```python
from build123d import *

# Parameters (mm, degrees)
SKETCH_W     = 80
SKETCH_H     = 9.5
PAD_DEPTH    = 10
SKETCH001_W  = 70
SKETCH001_H  = 25
POCKET_DEPTH = 6.3
SKETCH002_R  = 0.8
HOLE_DEPTH   = 10.001


with BuildPart() as part:
    # Sketch → Pad (new body)
    with BuildSketch(Plane.XY):
        with Locations((0, 2.25)):
            Rectangle(SKETCH_W, SKETCH_H)
    extrude(amount=PAD_DEPTH)

    # Sketch001 → Pocket (cut)
    with BuildSketch(Plane.XY):
        with Locations((0, -1.444008)):
            Rectangle(SKETCH001_W, SKETCH001_H)
    extrude(amount=POCKET_DEPTH, mode=Mode.SUBTRACT)

    # Sketch002 → Hole (cut, through all)
    with BuildSketch(Plane.XY):
        with Locations((37.5, 0)):
            Circle(SKETCH002_R)
        with Locations((-37.5, 0)):
            Circle(SKETCH002_R)
    extrude(amount=HOLE_DEPTH, mode=Mode.SUBTRACT)


solid = part.part
```
For this review, take the finished solid that the model builds, in its own axes (mm). A direction names the side the tool comes from. Coordinates: 2 decimals unless noted, no trailing zeros. Order: outer loops, then holes, each group sorted by start corner. A loop starts at its lowest first (then second) coordinate and runs counter-clockwise, first axis right, second up. Notation, with made-up numbers: (20, 73.25) - (30, 73.25) arc R19 ccw to (30, 85.25) - close; hole circle Ø4 at (-32.75, -4). An arc over 180 degrees is marked (long way). Answer as a JSON object with one key per item and string values. Group by question number.
1. Clearance check with a flat-ended pin moving along its axis: P1, Ø3, axis at x = 7.5, y = 3, coming from the -Z side. State where the tip first meets the part, or that it passes through.
2. For faces 4 (the flat face through (35, 2, 3)), 5 (the flat face through (-1, 2, 10)), list the 3-axis set-ups (+Z, -Z, +X, -X, +Y, -Y) from which the entire face can be reached by the end or side of a thin tool; tool diameter is ignored.
3. The part is to be moulded in two halves that separate along Y. For faces 1 (the flat face through (-35, 2, 3)), 2 (the flat face through (-9, -2.5, 7)), 3 (the cylindrical face through (38.263, 0.24, 4.93)), say which applies: pulls with the +Y half, pulls with the -Y half, needs draft (parallel to the pull), parting line crosses it, or undercut.
4. We need section A-A on x = -37.5. State the section outline as (y, z) points.
5. We need section B-B on y = 0. State the section outline as (x, z) points, then the cut area to 3 significant figures.
6. We need section C-C on x = -18. State the section outline as (y, z) points, then the cut area to 4 significant figures.
7. For probe 1 along X at (y, z) = (0, 7.75); probe 2 along Y at (x, z) = (37.5, 6.25); probe 3 along X at (y, z) = (0, 4.5), list the stretches that pass through material, from the lowest coordinate up.
Final values:
{
 "1": {"P1": "z = 6.3"},
 "2": {"face 4": "-Z, +Y, -Y", "face 5": "+Z, +X, -X, +Y, -Y"},
 "3": {"face 1": "needs draft", "face 2": "pulls with the -Y half", "face 3": "undercut"},
 "4": {"outline": "(-2.5, 0) - (-0.8, 0) - (-0.8, 10) - (-2.5, 10) - close; (0.8, 0) - (7, 0) - (7, 10) - (0.8, 10) - close"},
 "5": {"outline": "(-40, 0) - (-38.3, 0) - (-38.3, 10) - (-40, 10) - close; (-36.7, 0) - (-35, 0) - (-35, 6.3) - (35, 6.3) - (35, 0) - (36.7, 0) - (36.7, 10) - (-36.7, 10) - close; (38.3, 0) - (40, 0) - (40, 10) - (38.3, 10) - close", "area": "327 mm²"},
 "6": {"outline": "(-2.5, 6.3) - (7, 6.3) - (7, 10) - (-2.5, 10) - close", "area": "35.15 mm²"},
 "7": {"probe 1": "-40 to -38.3, -36.7 to 36.7, 38.3 to 40", "probe 2": "-2.5 to -0.8, 0.8 to 7", "probe 3": "-40 to -38.3, -36.7 to -35, 35 to 36.7, 38.3 to 40"}
}
